Input: part model. Units: mm. Frame: model coordinates. Face numbers are marked on the shaded views. A direction names the side the tool comes from. Coordinates: 2 decimals unless noted, no trailing zeros. Loops run counter-clockwise (first coordinate to the right, second up) from the corner with the lowest first, then second, coordinate; pieces in that order, holes last. Notation, with made-up numbers: M 65.25,46 L 70.25,46 A20 cw 70.25,78 Z; hole C 57.5,-40 d1. An arc over 180 degrees is marked long. Use a Markdown table: item, result. Add a question column.
1. Set-up query: the marked faces 1, 2 and 3. Return all of +Z, -Z, +X, -X, +Y, -Y with unobstructed straight access to the full face (end or side cutting, diameter ignored); none if empty.
2. Section B-B on y = 8.5. Output: boundary loops of the cut face in (x, z), then the cut area to 3 significant figures.
3. Line query: L1, parallel to Y at x = -10, z = 19.5; L2, parallel to Y at x = -6, z = -2.5; L3, parallel to Y at x = -19, z = 10.5. Output: solid intervals per line, ascending. Write a range as [from, to].
4. Section A-A on y = 26.5. Output: boundary loops of the cut face in (x, z), then the cut area to 3 significant figures.
5. Pin query (flat end, axial travel): pin 1 (1.9 mm diameter, centred on x = -10, y = 36, fed in from +Z); pin 2 (2.5 mm diameter, centred on x = 10, y = 36, fed in from +Z); pin 3 (7.5 mm diameter, centred on x = 0, z = -20, fed in from +Y); pin 4 (1.6 mm diameter, centred on y = 29.5, z = 14.5, fed in from +X). Return the tip coordinate at first contact, or that it passes through.
```python
from build123d import *

# Parameters (mm, degrees)
SKETCH1_W           = 141
SKETCH1_H           = 70
BOSS_EXTRUDE1_DEPTH = 2
SKETCH2_W           = 30
SKETCH2_H           = 2
BOSS_EXTRUDE2_DEPTH = 40
SKETCH3_R           = 1.05
CUT_EXTRUDE1_DEPTH  = 20
CHAMFER1_SIZE       = 5
CHAMFER2_SIZE       = 10
CHAMFER3_SIZE       = 4
CHAMFER4_SIZE       = 10
SKETCH4_R           = 3.175
CUT_EXTRUDE2_DEPTH  = 10
SKETCH5_R           = 4.974636633
SKETCH5_R_2         = 3.146236459
SKETCH5_R_3         = 4.54576988
SKETCH5_R_4         = 5.519543083
SKETCH5_R_5         = 4.37453593
SKETCH5_R_6         = 4.123519833
SKETCH5_R_7         = 4.733675758
SKETCH5_R_8         = 5.109952542
SKETCH5_R_9         = 4.930902715
SKETCH5_R_10        = 3.1185767
SKETCH5_R_11        = 4.186079964
SKETCH5_R_12        = 3.423196992
SKETCH5_R_13        = 5.083908884
SKETCH5_R_14        = 5.746414823
SKETCH5_R_15        = 4.82911997
SKETCH5_R_16        = 1.618250018
SKETCH5_R_17        = 1.536391082
SKETCH5_R_18        = 2.291759317
SKETCH5_R_19        = 3.534495501
SKETCH5_R_20        = 2.885901018
SKETCH5_R_21        = 2.983748602
SKETCH5_R_22        = 3.273704374
SKETCH5_R_23        = 1.749106038
SKETCH5_R_24        = 1.76916029
SKETCH5_R_25        = 2.701911231
SKETCH5_R_26        = 2.165520053
SKETCH5_R_27        = 2.467098103
SKETCH5_R_28        = 1.303971465
SKETCH5_R_29        = 2.25029129
CUT_EXTRUDE3_DEPTH  = 10


with BuildPart() as part:
    # Sketch1 → Boss-Extrude1 (new body)
    with BuildSketch(Plane(origin=(0, 0, 0), x_dir=(1, 0, 0), z_dir=(0, 1, 0))):
        Rectangle(SKETCH1_W, SKETCH1_H)
    extrude(amount=BOSS_EXTRUDE1_DEPTH)

    # Sketch2 → Boss-Extrude2 (add)
    with BuildSketch(Plane(origin=(0, 2, 0), x_dir=(1, 0, 0), z_dir=(0, 1, 0))):
        with Locations((0, -15)):
            Rectangle(SKETCH2_W, SKETCH2_H)
        with Locations((0, -19)):
            Rectangle(SKETCH2_W, SKETCH2_H)
    extrude(amount=BOSS_EXTRUDE2_DEPTH)

    # Sketch3 → Cut-Extrude1 (cut)
    with BuildSketch(Plane.XY.offset(20)):
        with Locations((-10, 16)):
            Circle(SKETCH3_R)
        with Locations((-10, 36)):
            Circle(SKETCH3_R)
        with Locations((10, 36)):
            Circle(SKETCH3_R)
        with Locations((10, 16)):
            Circle(SKETCH3_R)
    extrude(amount=-CUT_EXTRUDE1_DEPTH, mode=Mode.SUBTRACT)

    # Chamfer1
    chamfer1_edges = [part.edges().sort_by_distance(p)[0] for p in [
        (-15, 42, 15),
        (15, 42, 15),
        (-15, 42, 19),
        (15, 42, 19),
    ]]
    chamfer(chamfer1_edges, length=CHAMFER1_SIZE)

    # Chamfer2
    chamfer2_edges = [part.edges().sort_by_distance(p)[0] for p in [
        (-15, 2, 15),
        (15, 2, 15),
        (-15, 2, 19),
        (15, 2, 19),
    ]]
    chamfer(chamfer2_edges, length=CHAMFER2_SIZE)

    # Chamfer3
    chamfer3_edges = [part.edges().sort_by_distance(p)[0] for p in [
        (0, 2, 14),
        (0, 2, 20),
    ]]
    chamfer(chamfer3_edges, length=CHAMFER3_SIZE)

    # Chamfer4
    chamfer4_edges = [part.edges().sort_by_distance(p)[0] for p in [
        (70.5, 1, 35),
        (-70.5, 1, 35),
    ]]
    chamfer(chamfer4_edges, length=CHAMFER4_SIZE)

    # Sketch4 → Cut-Extrude2 (cut)
    with BuildSketch(Plane(origin=(0, 2, 0), x_dir=(1, 0, 0), z_dir=(0, 1, 0))):
        with Locations((0, 20)):
            Circle(SKETCH4_R)
    extrude(amount=-CUT_EXTRUDE2_DEPTH, mode=Mode.SUBTRACT)

    # Sketch5 → Cut-Extrude3 (cut)
    with BuildSketch(Plane(origin=(0, 2, 0), x_dir=(1, 0, 0), z_dir=(0, 1, 0))):
        with Locations((-32.885567752, 11.811746645)):
            Circle(SKETCH5_R)
        with Locations((-35.487274061, -2.237467426)):
            Circle(SKETCH5_R_2)
        with Locations((-45.894099299, 6.400197521)):
            Circle(SKETCH5_R_3)
        with Locations((-45.894099299, 20.865684602)):
            Circle(SKETCH5_R_4)
        with Locations((-30.283861442, 26.385227685)):
            Circle(SKETCH5_R_5)
        with Locations((-19.877036204, 20.137206835)):
            Circle(SKETCH5_R_6)
        with Locations((-17.171261642, 9.001903831)):
            Circle(SKETCH5_R_7)
        with Locations((-24.000556037, -0.884580145)):
            Circle(SKETCH5_R_8)
        with Locations((-33.509977266, -16.39074975)):
            Circle(SKETCH5_R_7)
        with Locations((-47.038850075, -8.377494316)):
            Circle(SKETCH5_R_9)
        with Locations((-53.907354732, -19.512797321)):
            Circle(SKETCH5_R_10)
        with Locations((-45.894099299, -26.173165473)):
            Circle(SKETCH5_R_11)
        with Locations((-34.758796294, -27.630121007)):
            Circle(SKETCH5_R_12)
        with Locations((-61.504337156, -5.994532687)):
            Circle(SKETCH5_R_13)
        with Locations((-61.504337156, 9.001903831)):
            Circle(SKETCH5_R_14)
        with Locations((-60.255518127, 24.260726668)):
            Circle(SKETCH5_R_15)
        with Locations((-50.439869179, 32.313192364)):
            Circle(SKETCH5_R_16)
        with Locations((-41.348329419, 30.694942345)):
            Circle(SKETCH5_R_17)
        with Locations((-19.877036204, 29.158551263)):
            Circle(SKETCH5_R_18)
        with Locations((-10.198688733, 27.526052754)):
            Circle(SKETCH5_R_19)
        with Locations((-9.053937957, 18.368046545)):
            Circle(SKETCH5_R_20)
        with Locations((-6.664193232, 9.001903831)):
            Circle(SKETCH5_R_21)
        with Locations((-9.053937957, 0)):
            Circle(SKETCH5_R_22)
        with Locations((-15.753516372, -4.422900726)):
            Circle(SKETCH5_R_23)
        with Locations((-44.229007261, -17.847705283)):
            Circle(SKETCH5_R_24)
        with Locations((-24.000556037, -30.544032073)):
            Circle(SKETCH5_R_25)
        with Locations((-12.69632679, -30.544032073)):
            Circle(SKETCH5_R_26)
        with Locations((-3.330184076, -30.544032073)):
            Circle(SKETCH5_R_27)
        with Locations((-9.053937957, -26.173165473)):
            Circle(SKETCH5_R_28)
        with Locations((-18.003807661, -27.842120842)):
            Circle(SKETCH5_R_29)
    cut_extrude3 = extrude(amount=-CUT_EXTRUDE3_DEPTH, mode=Mode.SUBTRACT)

    # Mirror1: Cut-Extrude3 across plane
    add(cut_extrude3.mirror(Plane(origin=(0, 0, 0), x_dir=(0, 0, 1), z_dir=(1, 0, 0))), mode=Mode.SUBTRACT)


solid = part.part
```
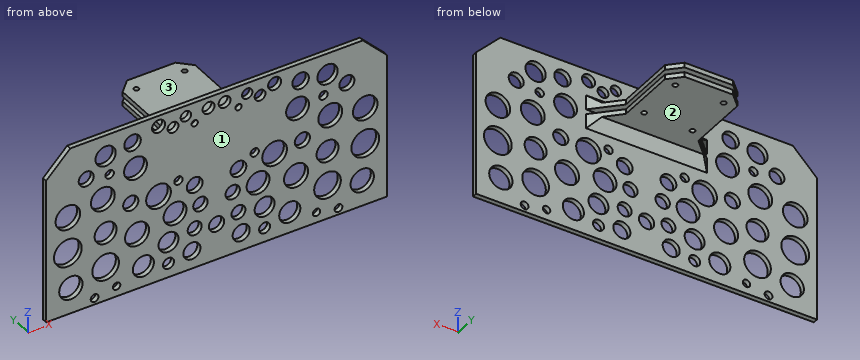
Answers below:
| question | item | result |
|---|---|---|
| 1 | face 1 | +Z, -Z, +X, -X, -Y |
| 1 | face 2 | -Z, +X, -X, +Y |
| 1 | face 3 | +Z, +X, -X, +Y |
| 2 | outline | M -18.5,14 L 18.5,14 L 18.5,16 L -18.5,16 Z; M -18.5,18 L 18.5,18 L 18.5,20 L -18.5,20 Z |
| 2 | area | 148 mm² |
| 3 | L1 | y = [0, 14.95], [17.05, 34.95], [37.05, 42] |
| 3 | L2 | y = [0, 2] |
| 3 | L3 | y = [0, 2.5] |
| 4 | outline | M -15,14 L 15,14 L 15,16 L -15,16 Z; M -15,18 L 15,18 L 15,20 L -15,20 Z |
| 4 | area | 120 mm² |
| 5 | pin 1 | passes through |
| 5 | pin 2 | stops at z = 20 |
| 5 | pin 3 | stops at y = 2 |
| 5 | pin 4 | stops at x = 15 |
